Check sheet for the modelled part. Datum: model origin and axes. Units: mm. A direction names the side the tool comes from. Give positions to 0.01 mm unless a question says otherwise; leave off trailing zeros. Order: outer loops, then holes, each group sorted by start corner. A loop starts at its lowest first (then second) coordinate and runs counter-clockwise, first axis right, second up. Notation, with made-up numbers: (11, -3.5) - (33, -3.5) arc R32 cw to (33, 35.5) - close; hole circle Ø11 at (-13.75, -24). An arc over 180 degrees is marked (long way). Answer in a Markdown table with one row per item.
from build123d import *

# Parameters (mm, degrees)
F1_DEPTH = 70
F2_W     = 40
F2_H     = 20
F3_DEPTH = 130.001
F4_R     = 5
F5_W     = 30
F5_H     = 30
F6_DEPTH = 20


with BuildPart() as f1:
    # F0 (on Front) → F1 (new body)
    with BuildSketch(Plane.XZ):
        Polygon((65, 35), (15, 35), (-25, -5), (-65, -5), (-65, -35), (65, -35), align=None)
    extrude(amount=F1_DEPTH)

    # F2 (on face) → F3 (cut, through all)
    with BuildSketch(Plane.YZ.offset(65)):
        with Locations((-35, 15)):
            Rectangle(F2_W, F2_H)
    extrude(amount=-F3_DEPTH, mode=Mode.SUBTRACT)

    # F4
    f4_edges = [f1.edges().sort_by_distance(p)[0] for p in [
        (25, -55, 5),
        (25, -15, 5),
        (35, -15, 25),
        (35, -55, 25),
    ]]
    fillet(f4_edges, radius=F4_R)

    # F5 (on face) → F6 (cut)
    with BuildSketch(Plane(origin=(-65, 0, 0), x_dir=(0, -1, 0), z_dir=(-1, 0, 0))):
        with Locations((35, -20)):
            Rectangle(F5_W, F5_H)
    extrude(amount=-F6_DEPTH, mode=Mode.SUBTRACT)


solid = f1.part
(1) Mould release check, pull along Y, two halves, no side actions. Record for faces 4 (the flat face through (-44.7, -34.5, -5)), 5 (the flat face through (-45, -35, -20)), 6 (the flat face through (14, -70, -7)): pulls with the +Y half, pulls with the -Y half, needs draft (parallel to the pull), parting line crosses it, or undercut.
Geometry says:
| item | result |
|---|---|
| face 4 | needs draft |
| face 5 | undercut |
| face 6 | pulls with the -Y half |
(2) Thickness scan on L1, parallel to Y at x = -46.5, z = -13; L2, parallel to Z at x = 51.5, y = -41; L3, parallel to Y at x = 2.5, z = 19.5. Record the ranges inside material, lowest first.
Geometry says:
| item | result |
|---|---|
| L1 | -70 to -50, -20 to 0 |
| L2 | -35 to 5, 25 to 35 |
| L3 | -70 to -55, -15 to 0 |
(3) Cross-section at A-A, the plane z = 23. Record the cut outline in (x, y), then the cut area to 3 significant figures.
Geometry says:
| item | result |
|---|---|
| outline | (3, -70) - (65, -70) - (65, -54) - (3, -54) - close; (3, -16) - (65, -16) - (65, 0) - (3, 0) - close |
| area | 1,980 mm² |
(4) Cross-section at C-C, the plane x = 55. Record the cut outline in (y, z), then the cut area to 3 significant figures.
Geometry says:
| item | result |
|---|---|
| outline | (-70, -35) - (0, -35) - (0, 35) - (-70, 35) - close; hole (-55, 10) arc R5 ccw to (-50, 5) - (-20, 5) arc R5 ccw to (-15, 10) - (-15, 20) arc R5 ccw to (-20, 25) - (-50, 25) arc R5 ccw to (-55, 20) - close |
| area | 4,120 mm² |
(5) Cross-section at D-D, the plane x = -13. Record the cut outline in (y, z).
Geometry says:
| item | result |
|---|---|
| outline | (-70, -35) - (0, -35) - (0, 7) - (-16, 7) arc R5 cw to (-20, 5) - (-50, 5) arc R5 cw to (-54, 7) - (-70, 7) - close |
(6) Access from +Z, -Z, +X, -X, +Y, -Y to the whole of each face (thin tool, end or side, straight path). Record for faces 1 (the flat face through (-55, -50, -20)), 2 (the flat face through (-65, -10, -20)), 3 (the cylindrical face through (24, -54, 7)).
Geometry says:
| item | result |
|---|---|
| face 1 | +Z, -Z, -X |
| face 2 | +Z, -Z, -X, +Y, -Y |
| face 3 | +X, -X |
(7) Gauge pin test, flat end, axial feed: P1, Ø5, axis at y = -28, z = -11.5, coming from the -X side. Record the tip position at first contact, or that the pin passes through.
Geometry says:
| item | result |
|---|---|
| P1 | x = -45 |
(8) Cross-section at B-B, the plane y = -29. Record the cut outline in (x, z), then the cut area to 3 significant figures.
Geometry says:
| item | result |
|---|---|
| outline | (-45, -35) - (65, -35) - (65, 5) - (-15, 5) - (-25, -5) - (-45, -5) - close; (5, 25) - (65, 25) - (65, 35) - (15, 35) - close |
| area | 4,700 mm² |
